```python
from build123d import *

# Parameters (mm, degrees)
F0_W      = 71.4248
F0_H      = 123.825
F1_DEPTH  = 25.4
F2_W      = 63.5
F2_H      = 44.45
F3_DEPTH  = 22.225
F4_W      = 4.7625
F4_H      = 25.4
F5_DEPTH  = 4.7625
F6_W      = 4.7625
F6_H      = 25.4
F7_DEPTH  = 4.7625
F9_DEPTH  = 19.05
F11_DEPTH = 19.05
F12_R     = 12.7
F12_W     = 12.7
F12_H     = 34.925
F13_DEPTH = 6.35
F14_R     = 6.35
F15_DEPTH = 25.4
F16_R     = 6.35
F17_DEPTH = 25.4


with BuildPart() as f1:
    # F0 (on Top) → F1 (new body)
    with BuildSketch(Plane.XY):
        with Locations((2.37449, 5.994919)):
            Rectangle(F0_W, F0_H)
    extrude(amount=F1_DEPTH)

    # F2 (on face) → F3 (cut)
    with BuildSketch(Plane.XY.offset(25.4)):
        with Locations((2.24492, 32.982419)):
            Rectangle(F2_W, F2_H)
        with Locations((2.24492, -20.992581)):
            Rectangle(F2_W, F2_H)
    extrude(amount=-F3_DEPTH, mode=Mode.SUBTRACT)

    # F4 (on face) → F5 (cut)
    with BuildSketch(Plane.YZ.offset(38.08689)):
        with Locations((62.351169, 12.7)):
            Rectangle(F4_W, F4_H)
        with Locations((-50.361331, 12.7)):
            Rectangle(F4_W, F4_H)
    extrude(amount=-F5_DEPTH, mode=Mode.SUBTRACT)

    # F6 (on face) → F7 (cut)
    with BuildSketch(Plane(origin=(-33.33791, 0, 0), x_dir=(0, -1, 0), z_dir=(-1, 0, 0))):
        with Locations((-62.351169, 12.7)):
            Rectangle(F6_W, F6_H)
        with Locations((50.361331, 12.7)):
            Rectangle(F6_W, F6_H)
    extrude(amount=-F7_DEPTH, mode=Mode.SUBTRACT)

    # F8 (on face) → F9 (cut)
    with BuildSketch(Plane(origin=(0, 0, 0), x_dir=(1, 0, 0), z_dir=(0, 0, -1))):
        Polygon((-33.33791, -67.907419), (38.08689, -67.907419), (38.08689, -64.732419), (33.32439, -64.732419), (33.32439, -59.969919), (38.08689, -59.969919), (38.08689, -58.382419), (-33.33791, -58.382419), (-33.33791, -59.969919), (-28.57541, -59.969919), (-28.57541, -64.732419), (-33.33791, -64.732419), align=None)
    extrude(amount=-F9_DEPTH, mode=Mode.SUBTRACT)

    # F10 (on face) → F11 (cut)
    with BuildSketch(Plane(origin=(0, 0, 0), x_dir=(1, 0, 0), z_dir=(0, 0, -1))):
        Polygon((38.08689, 52.742581), (38.08689, 55.917581), (-33.33791, 55.917581), (-33.33791, 52.742581), (-28.57541, 52.742581), (-28.57541, 47.980081), (-33.33791, 47.980081), (-33.33791, 46.392581), (38.08689, 46.392581), (38.08689, 47.980081), (33.32439, 47.980081), (33.32439, 52.742581), align=None)
    extrude(amount=-F11_DEPTH, mode=Mode.SUBTRACT)

    # F12 (on face) → F13 (cut)
    with BuildSketch(Plane.XY.offset(3.175)):
        with Locations((-13.63008, 39.332419)):
            Circle(F12_R)
        with Locations((24.46992, 32.982419)):
            Rectangle(F12_W, F12_H)
        with Locations((-19.98008, -20.992581)):
            Rectangle(F12_W, F12_H)
        with Locations((18.11992, -27.342581)):
            Circle(F12_R)
    extrude(amount=-F13_DEPTH, mode=Mode.SUBTRACT)

    # F14 (on face) → F15 (cut)
    with BuildSketch(Plane.XZ.offset(-55.207419)):
        with Locations((21.29492, 14.2875)):
            Circle(F14_R)
    extrude(amount=-F15_DEPTH, mode=Mode.SUBTRACT)

    # F16 (on face) → F17 (cut)
    with BuildSketch(Plane(origin=(0, -43.217581, 0), x_dir=(-1, 0, 0), z_dir=(0, 1, 0))):
        with Locations((16.80508, 14.2875)):
            Circle(F16_R)
    extrude(amount=-F17_DEPTH, mode=Mode.SUBTRACT)


solid = f1.part
```
The model under review builds one solid part; all positions refer to its coordinate system, in mm. A direction names the side the tool comes from. Round coordinates to 2 decimals unless told otherwise and drop trailing zeros. Loops run counter-clockwise (first coordinate to the right, second up) from the corner with the lowest first, then second, coordinate; pieces in that order, holes last.
1) Clearance check with flat-ended pins moving along their axes: P1, Ø1.5, axis at x = 29, z = 16.5, coming from the -Y side; P2, Ø2, axis at x = 2, y = 52, coming from the +Z side (3 decimals); P3, Ø7.5, axis at x = 34, y = 64, coming from the -Z side. State where each tip first meets the part, or that it passes through.
Values follow:
P1: stops at y = -46.39
P2: stops at z = 3.175
P3: stops at z = 19.05
2) Wall thickness on line 1 along Y through (x, z) = (33.5, 9.75); line 2 along Y through (x, z) = (4, 21); line 3 along X through (y, z) = (35, 17.25): over which ranges is each line inside the solid? List them lowest first.
Values follow:
line 1: y = -46.39 to -43.22, 1.23 to 10.76, 55.21 to 58.38
line 2: y = -55.92 to -43.22, 1.23 to 10.76, 55.21 to 67.91
line 3: x = -33.34 to -29.51, 33.99 to 38.09
3) Consider section B-B on z = 5. State the section outline as (x, y) points, then the cut area to 3 significant figures.
Values follow:
outline: (-33.34, -46.39) - (38.09, -46.39) - (38.09, 58.38) - (-33.34, 58.38) - close; hole (-29.51, -43.22) - (33.99, -43.22) - (33.99, 1.23) - (-29.51, 1.23) - close; hole (-29.51, 10.76) - (33.99, 10.76) - (33.99, 55.21) - (-29.51, 55.21) - close
area: 1,840 mm2
4) Consider section A-A on y = -11.5. State the section outline as (x, z) points (3 decimals).
Values follow:
outline: (-33.338, 0) - (-26.33, 0) - (-26.33, 3.175) - (-29.505, 3.175) - (-29.505, 25.4) - (-33.338, 25.4) - close; (-13.63, 0) - (38.087, 0) - (38.087, 25.4) - (33.995, 25.4) - (33.995, 3.175) - (-13.63, 3.175) - close
5) Consider section D-D on x = 9. State the section outline as (y, z) points (3 decimals).
Values follow:
outline: (-55.918, 19.05) - (-46.393, 19.05) - (-46.393, 0) - (-36.181, 0) - (-36.181, 3.175) - (-43.218, 3.175) - (-43.218, 25.4) - (-55.918, 25.4) - close; (-18.504, 0) - (58.382, 0) - (58.382, 19.05) - (67.907, 19.05) - (67.907, 25.4) - (55.207, 25.4) - (55.207, 3.175) - (10.757, 3.175) - (10.757, 25.4) - (1.232, 25.4) - (1.232, 3.175) - (-18.504, 3.175) - close
6) Consider section C-C on x = -19.5. State the section outline as (y, z) points (3 decimals), then the cut area to 3 significant figures.
Values follow:
outline: (-55.918, 20.037) - (-43.218, 20.037) - (-43.218, 25.4) - (-55.918, 25.4) - close; (-46.393, 0) - (-38.455, 0) - (-38.455, 3.175) - (-43.218, 3.175) - (-43.218, 8.538) - (-46.393, 8.538) - close; (-3.53, 0) - (28.07, 0) - (28.07, 3.175) - (10.757, 3.175) - (10.757, 25.4) - (1.232, 25.4) - (1.232, 3.175) - (-3.53, 3.175) - close; (50.594, 0) - (58.382, 0) - (58.382, 19.05) - (67.907, 19.05) - (67.907, 25.4) - (55.207, 25.4) - (55.207, 3.175) - (50.594, 3.175) - close
area: 578 mm2
7) The part is to be moulded in two halves that separate along Z. For faces 5 (the face through (20.468, 58.646, 20.583)), 6 (the face through (2, -55.918, 22)), 7 (the face through (2, 6, 25.4)), say which applies: pulls with the +Z half, pulls with the -Z half, needs draft (parallel to the pull), parting line crosses it, or undercut.
Values follow:
face 5: undercut
face 6: needs draft
face 7: pulls with the +Z half
8) Tool access review of faces 1 (the face through (3, 58.382, 9)), 2 (the face through (33.324, 62, 22)), 3 (the face through (24, 15.52, 2)), 4 (the face through (2, 1.232, 14)): name each direction out of +Z, -Z, +X, -X, +Y, -Y from which nothing blocks a thin tool from reaching the whole face with its end or side.
Values follow:
face 1: -Z, +X, -X, +Y
face 2: +Z, -Z, +X
face 3: +Z, -Z
face 4: +Z
